Could you check a few things on this drawing? It's one solid part, dimensions in mm from its lowest x, y, z. Coordinates: 2 decimals unless noted, no trailing zeros. Write each loop counter-clockwise with the first axis right and the second up, starting at its lowest first coordinate (ties: lowest second). Pieces come first, ordered by that corner, then holes.
Item 1: I want a section at C-C (z = 18). Please give me the cut outline in (x, y), and give its area (3 significant figures).
Item 2: If we mould it in two halves opening along Y, with no side actions, what happens to the marked faces 1 and 2? For each: pulls with the +Y half, pulls with the -Y half, needs draft (parallel to the pull), parting line crosses it, or undercut.
Item 3: I want a section at A-A (y = 10.25). Please give me the cut outline in (x, z), and give its area (3 significant figures).
Item 4: I'm going to push flat-ended pins straight in: P1, Ø4, axis at x = 25.5, y = 14, coming from the -Z side; P2, Ø1, axis at x = 44.5, z = 18.5, coming from the -Y side; P3, Ø8, axis at x = 37.5, y = 19, coming from the -Z side. Where does each tip first touch, or does it pass through?
Item 5: Please list where these lines run through material, in increasing order: line 1 (Z direction, x = 35, y = 5.25); line 2 (Y direction, x = 44, z = 18); line 3 (Z direction, x = 3.5, y = 3.5).
Item 6: I want a section at D-D (y = 3). Please give me the cut outline in (x, z).
Item 7: I want a section at B-B (x = 47). Please give me the cut outline in (y, z), and give its area (3 significant figures).
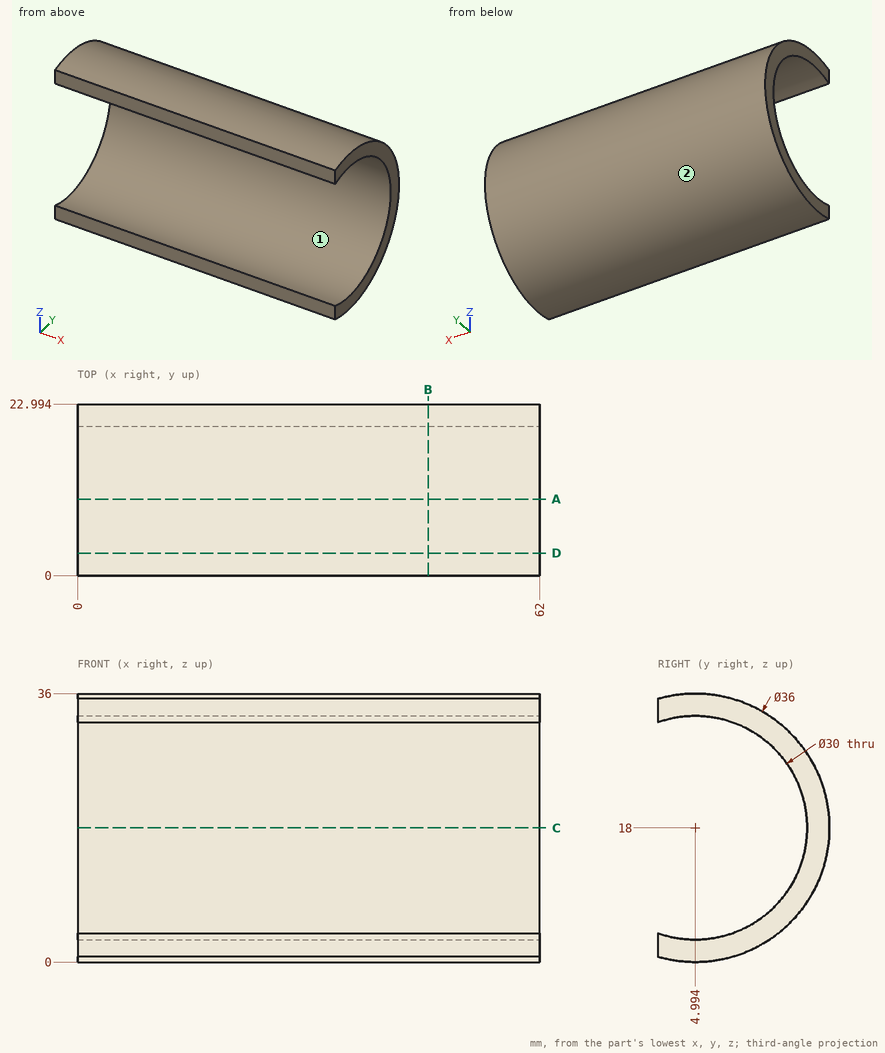
Answer:
1. outline: (0, 19.99) - (62, 19.99) - (62, 22.99) - (0, 22.99) - close
1. area: 186 mm2
2. face 1: undercut
2. face 2: parting line crosses it
3. outline: (0, 0.78) - (62, 0.78) - (62, 3.95) - (0, 3.95) - close; (0, 32.05) - (62, 32.05) - (62, 35.22) - (0, 35.22) - close
3. area: 393 mm2
4. P1: stops at z = 1.42
4. P2: stops at y = 19.96
4. P3: stops at z = 3.04
5. line 1: z = 0 to 3, 33 to 36
5. line 2: y = 19.99 to 22.99
5. line 3: z = 0.06 to 3.07, 32.93 to 35.94
6. outline: (0, 0.11) - (62, 0.11) - (62, 3.13) - (0, 3.13) - close; (0, 32.87) - (62, 32.87) - (62, 35.89) - (0, 35.89) - close
7. outline: (0, 0.71) arc R18 ccw (long way) to (0, 35.29) - (0, 32.14) arc R15 cw (long way) to (0, 3.86) - close
7. area: 186 mm2
